Work out the finished part from the listing and answer in its coordinate system (mm). Give positions to 0.01 mm unless a question says otherwise; leave off trailing zeros. Loops run counter-clockwise (first coordinate to the right, second up) from the corner with the lowest first, then second, coordinate; pieces in that order, holes last. Notation, with made-up numbers: M 28,75 L 42,75 A13 cw 42,85 Z; hole C 89,12 d7. An arc over 180 degrees is marked long. Use a Markdown table: item, result.
Autodesk Inventor part; units mm, degrees
ref_plane "YZ Plane" through (0, 0, 0) normal (1, 0, 0) x (0, 1, 0)
ref_plane "XZ Plane" through (0, 0, 0) normal (0, 1, 0) x (-1, 0, 0)
ref_plane "XY Plane" through (0, 0, 0) normal (0, 0, 1) x (1, 0, 0)
sketch "Sketch1" plane through (0, 0, 0) normal (0, 0, 1) x (1, 0, 0)
  arc A0 (0, -30) -> (0, 30) centre (0, 0) ccw
  line L0 (0, 0) -> (300, 0)
  arc A1 (300, 30) -> (300, -30) centre (300, 0) ccw
  line L1 (300, 30) -> (0, 30)
  line L2 (300, -30) -> (0, -30)
  dimension "d6" = 60
  dimension "d7" = 300
  dimension "d8" = 60
extrude "Extrusion2" add sketch "Sketch1" along normal blind 20
fillet "Fillet2" radius 3 4 edges at (300, 30, 10) (300, -30, 10) (0, -30, 10) (0, 30, 10)
properties part number "arm_0_extension_attacher"
(1) Consider probe 1 along X at (y, z) = (-12, 14.25); probe 2 along X at (y, z) = (3.5, 10.25). Determine where each line is inside the solid, lowest interval first. Write a range as [from, to].
Entries:
| item | result |
|---|---|
| probe 1 | x = [27.5, 272.5] |
| probe 2 | x = [29.8, 270.2] |
(2) A cutting plane is placed at B-B (y = -14). Write down the section's boundary in (x, z).
Entries:
| item | result |
|---|---|
| outline | M 26.53,0 L 273.47,0 L 273.47,20 L 26.53,20 Z |
(3) A cutting plane is placed at A-A (y = 21.5). Write down the section's boundary in (x, z), and give its area (3 significant figures).
Entries:
| item | result |
|---|---|
| outline | M 20.92,0 L 279.08,0 L 279.08,20 L 20.92,20 Z |
| area | 5,160 mm² |
(4) Given P1, Ø5, axis at y = -19, z = 13.5, coming from the +X side; P2, Ø8, axis at y = -4, z = 16, coming from the -X side; P3, Ø8, axis at y = -17, z = 17, coming from the +X side, each flat-ended and moving along its own axis, determine where each tip first touches the part or whether it passes through.
Entries:
| item | result |
|---|---|
| P1 | stops at x = 279.08 |
| P2 | stops at x = 28.91 |
| P3 | stops at x = 278.58 |
